The figure shows three views and two pictorial views of one solid part (mm, origin at its lowest corner). Answer the questions. Coordinates: 2 decimals unless noted, no trailing zeros. Loops run counter-clockwise (first coordinate to the right, second up) from the corner with the lowest first, then second, coordinate; pieces in that order, holes last. Notation, with made-up numbers: M 62.5,72 L 92.5,72 A32 cw 92.5,110 Z; hole C -29,-32 d2. An arc over 180 degrees is marked long. One line per item, written item: value. Start each with the question number.
1. Consider probe 1 along Y at (x, z) = (31, 29.5); probe 2 along Z at (x, y) = (273, 96); probe 3 along Z at (x, y) = (328, 28). Determine where each line is inside the solid, lowest interval first.
2. Flat-ended cylindrical pins translate along their axes: pin 1 (1.5 mm diameter, centred on x = 321, z = 41.5, fed in from -Y); pin 2 (1.5 mm diameter, centred on x = 496.5, y = 14, fed in from -Z); pin 3 (4 mm diameter, centred on x = 208, z = 22.5, fed in from +Y). Find the tip coordinate at first contact, or state that the pin passes through.
3. The part is cut by section A-A (x = 255). Write down the section's boundary in (y, z), then the cut area to 3 significant figures.
4. The part is cut by section C-C (z = 20.5). Write down the section's boundary in (x, y), then the cut area to 3 significant figures.
5. The part is cut by section B-B (y = 117). Write down the section's boundary in (x, z), then the cut area to 3 significant figures.
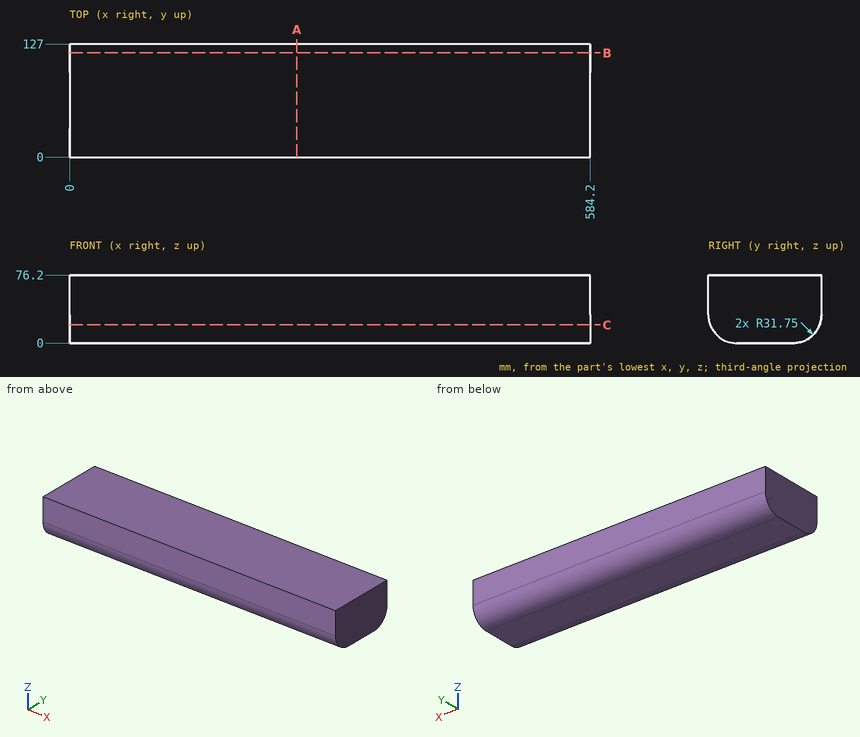
Answer block:
1. probe 1: y = 0.08 to 126.92
1. probe 2: z = 0.01 to 76.2
1. probe 3: z = 0.22 to 76.2
2. pin 1: stops at y = 0
2. pin 2: stops at z = 4.93
2. pin 3: stops at y = 126.16
3. outline: M 0,31.75 A31.75 ccw 31.75,0 L 95.25,0 A31.75 ccw 127,31.75 L 127,76.2 L 0,76.2 Z
3. area: 9,240 mm2
4. outline: M 0,2.06 L 584.2,2.06 L 584.2,124.94 L 0,124.94 Z
4. area: 71,800 mm2
5. outline: M 0,8.62 L 584.2,8.62 L 584.2,76.2 L 0,76.2 Z
5. area: 39,500 mm2
